```python
from build123d import *

# Parameters (mm, degrees)
CROQUIS1_W                 = 140
CROQUIS1_H                 = 140
CROQUIS1_R                 = 1.5
SALIENTE_EXTRUIR1_DEPTH    = 50
CROQUIS2_R                 = 1.75
CROQUIS2_W                 = 50
CROQUIS2_H                 = 50
CORTAR_EXTRUIR1_DEPTH      = 143
CROQUIS3_W                 = 144
CROQUIS3_H                 = 144
CROQUIS3_R                 = 1.75
CROQUIS3_W_2               = 50
CROQUIS3_H_2               = 50
SALIENTE_EXTRUIR3_DEPTH    = 50
CORTAR_EXTRUIR2_REACH      = 170.582
CORTAR_EXTRUIR3_DEPTH      = 92
CORTAR_EXTRUIR3_DEPTH_BACK = 78


with BuildPart() as part:
    # Croquis1 → Saliente-Extruir1 (new body)
    with BuildSketch(Plane(origin=(0, 0, 0), x_dir=(1, 0, 0), z_dir=(0, 1, 0))):
        Rectangle(CROQUIS1_W, CROQUIS1_H)
        with Locations(Location((-61, 61, 0), (0, 0, 270))):
            Circle(CROQUIS1_R, mode=Mode.SUBTRACT)
        with Locations(Location((66, 61, 0), (0, 0, 270))):
            Circle(CROQUIS1_R, mode=Mode.SUBTRACT)
        with Locations(Location((66, -61, 0), (0, 0, 270))):
            Circle(CROQUIS1_R, mode=Mode.SUBTRACT)
        with Locations(Location((-61, -61, 0), (0, 0, 270))):
            Circle(CROQUIS1_R, mode=Mode.SUBTRACT)
        with Locations(Location((66, 30.5, 0), (0, 0, 270))):
            Circle(CROQUIS1_R, mode=Mode.SUBTRACT)
        with Locations(Location((66, -30.5, 0), (0, 0, 270))):
            Circle(CROQUIS1_R, mode=Mode.SUBTRACT)
        with Locations(Location((-30.5, -66, 0), (0, 0, 270))):
            Circle(CROQUIS1_R, mode=Mode.SUBTRACT)
        with Locations(Location((30.5, -66, 0), (0, 0, 270))):
            Circle(CROQUIS1_R, mode=Mode.SUBTRACT)
        with Locations(Location((-30.5, 66, 0), (0, 0, 90))):
            Circle(CROQUIS1_R, mode=Mode.SUBTRACT)
        with Locations(Location((30.5, 66, 0), (0, 0, 90))):
            Circle(CROQUIS1_R, mode=Mode.SUBTRACT)
        with Locations(Location((-66, 30.5, 0), (0, 0, 90))):
            Circle(CROQUIS1_R, mode=Mode.SUBTRACT)
        with Locations(Location((-66, -30.5, 0), (0, 0, 90))):
            Circle(CROQUIS1_R, mode=Mode.SUBTRACT)
    extrude(amount=SALIENTE_EXTRUIR1_DEPTH)

    # Croquis2 → Cortar-Extruir1 (cut)
    with BuildSketch(Plane(origin=(0, 50, 0), x_dir=(1, 0, 0), z_dir=(0, 1, 0))):
        with Locations(Location((66, 61, 0), (0, 0, 270))):
            Circle(CROQUIS2_R)
        with Locations(Location((-61, 61, 0), (0, 0, 270))):
            Circle(CROQUIS2_R)
        with Locations(Location((-61, -61, 0), (0, 0, 270))):
            Circle(CROQUIS2_R)
        with Locations(Location((66, -61, 0), (0, 0, 270))):
            Circle(CROQUIS2_R)
        Polygon((-28.906513257, 63.24), (-27.313026514, 66), (-28.906513257, 68.76), (-32.093486743, 68.76), (-33.686973486, 66), (-32.093486743, 63.24), align=None)
        Polygon((32.093486743, 63.24), (33.686973486, 66), (32.093486743, 68.76), (28.906513257, 68.76), (27.313026514, 66), (28.906513257, 63.24), align=None)
        Polygon((67.593486743, 27.74), (69.186973486, 30.5), (67.593486743, 33.26), (64.406513257, 33.26), (62.813026514, 30.5), (64.406513257, 27.74), align=None)
        Polygon((67.593486743, -33.26), (69.186973486, -30.5), (67.593486743, -27.74), (64.406513257, -27.74), (62.813026514, -30.5), (64.406513257, -33.26), align=None)
        Polygon((32.093486743, -68.76), (33.686973486, -66), (32.093486743, -63.24), (28.906513257, -63.24), (27.313026514, -66), (28.906513257, -68.76), align=None)
        Polygon((-28.906513257, -68.76), (-27.313026514, -66), (-28.906513257, -63.24), (-32.093486743, -63.24), (-33.686973486, -66), (-32.093486743, -68.76), align=None)
        Polygon((-64.406513257, -33.26), (-62.813026514, -30.5), (-64.406513257, -27.74), (-67.593486743, -27.74), (-69.186973486, -30.5), (-67.593486743, -33.26), align=None)
        Polygon((-64.406513257, 27.74), (-62.813026514, 30.5), (-64.406513257, 33.26), (-67.593486743, 33.26), (-69.186973486, 30.5), (-67.593486743, 27.74), align=None)
        Rectangle(CROQUIS2_W, CROQUIS2_H)
    extrude(amount=-CORTAR_EXTRUIR1_DEPTH, mode=Mode.SUBTRACT)

    # Croquis3 → Saliente-Extruir3 (add)
    with BuildSketch(Plane(origin=(0, 50, 0), x_dir=(1, 0, 0), z_dir=(0, 1, 0))):
        Rectangle(CROQUIS3_W, CROQUIS3_H)
        with Locations(Location((-61, -61, 0), (0, 0, 270))):
            Circle(CROQUIS3_R, mode=Mode.SUBTRACT)
        with Locations(Location((-61, 61, 0), (0, 0, 270))):
            Circle(CROQUIS3_R, mode=Mode.SUBTRACT)
        with Locations(Location((66, 61, 0), (0, 0, 270))):
            Circle(CROQUIS3_R, mode=Mode.SUBTRACT)
        with Locations(Location((66, -61, 0), (0, 0, 270))):
            Circle(CROQUIS3_R, mode=Mode.SUBTRACT)
        Rectangle(CROQUIS3_W_2, CROQUIS3_H_2, mode=Mode.SUBTRACT)
        Polygon((-33.686973486, -66), (-32.093486743, -68.76), (-28.906513257, -68.76), (-27.313026514, -66), (-28.906513257, -63.24), (-32.093486743, -63.24), align=None, mode=Mode.SUBTRACT)
        Polygon((-67.593486743, -33.26), (-64.406513257, -33.26), (-62.813026514, -30.5), (-64.406513257, -27.74), (-67.593486743, -27.74), (-69.186973486, -30.5), align=None, mode=Mode.SUBTRACT)
        Polygon((28.906513257, 63.24), (32.093486743, 63.24), (33.686973486, 66), (32.093486743, 68.76), (28.906513257, 68.76), (27.313026514, 66), align=None, mode=Mode.SUBTRACT)
        Polygon((-33.686973486, 66), (-32.093486743, 63.24), (-28.906513257, 63.24), (-27.313026514, 66), (-28.906513257, 68.76), (-32.093486743, 68.76), align=None, mode=Mode.SUBTRACT)
        Polygon((62.813026514, 30.5), (64.406513257, 27.74), (67.593486743, 27.74), (69.186973486, 30.5), (67.593486743, 33.26), (64.406513257, 33.26), align=None, mode=Mode.SUBTRACT)
        Polygon((67.593486743, -33.26), (69.186973486, -30.5), (67.593486743, -27.74), (64.406513257, -27.74), (62.813026514, -30.5), (64.406513257, -33.26), align=None, mode=Mode.SUBTRACT)
        Polygon((33.686973486, -66), (32.093486743, -63.24), (28.906513257, -63.24), (27.313026514, -66), (28.906513257, -68.76), (32.093486743, -68.76), align=None, mode=Mode.SUBTRACT)
        Polygon((-64.406513257, 27.74), (-62.813026514, 30.5), (-64.406513257, 33.26), (-67.593486743, 33.26), (-69.186973486, 30.5), (-67.593486743, 27.74), align=None, mode=Mode.SUBTRACT)
    extrude(amount=-SALIENTE_EXTRUIR3_DEPTH)

    # Cortar-Extruir2: up to this face of the body (flat: up to its plane)
    cortar_extruir2_end = Plane(part.part.faces().sort_by_distance((72, 25, 0))[0])
    # Croquis4 → Cortar-Extruir2 (cut, up to the picked face)
    with BuildSketch(Plane.ZY.offset(72), mode=Mode.PRIVATE) as cortar_extruir2_sk1:
        Polygon((-25, 50), (-72, 3), (-72, 50), align=None)
    cortar_extruir2_tool1 = split(extrude(cortar_extruir2_sk1.sketch, amount=-CORTAR_EXTRUIR2_REACH, mode=Mode.PRIVATE), bisect_by=cortar_extruir2_end, keep=Keep.BOTH, mode=Mode.PRIVATE)
    # Croquis4 → Cortar-Extruir2 (cut, up to the picked face)
    with BuildSketch(Plane.ZY.offset(72), mode=Mode.PRIVATE) as cortar_extruir2_sk2:
        Polygon((72, 3), (72, 50), (25, 50), align=None)
    cortar_extruir2_tool2 = split(extrude(cortar_extruir2_sk2.sketch, amount=-CORTAR_EXTRUIR2_REACH, mode=Mode.PRIVATE), bisect_by=cortar_extruir2_end, keep=Keep.BOTH, mode=Mode.PRIVATE)
    add(cortar_extruir2_tool1.solids().sort_by(Axis((-72, 34.333333, -56.333333), (1, 0, 0)))[0], mode=Mode.SUBTRACT)
    add(cortar_extruir2_tool2.solids().sort_by(Axis((-72, 34.333333, 56.333333), (1, 0, 0)))[0], mode=Mode.SUBTRACT)

    # Croquis5 → Cortar-Extruir3 (cut, two sides: drawn at the far end of the back side and taken through both)
    with BuildSketch(Plane.XY.offset(-CORTAR_EXTRUIR3_DEPTH_BACK)):
        Polygon((-25, 50), (-72, 3), (-72, 50), align=None)
        Polygon((25, 50), (72, 3), (72, 50), align=None)
    extrude(amount=CORTAR_EXTRUIR3_DEPTH + CORTAR_EXTRUIR3_DEPTH_BACK, mode=Mode.SUBTRACT)


solid = part.part
```
Geometry: final body of the model. Coordinates: model frame, mm. A direction names the side the tool comes from. Round coordinates to 2 decimals unless told otherwise and drop trailing zeros. Loops run counter-clockwise (first coordinate to the right, second up) from the corner with the lowest first, then second, coordinate; pieces in that order, holes last. Notation, with made-up numbers: (39, -28) -> (63, -28) arc R24 ccw to (63, 2) -> close; hole circle Ø5 at (86.5, 27.25). An arc over 180 degrees is marked (long way). Write each question's results on one line, items separated by ' | '.
Item 1: Pull-direction query (Z, two-part tool) for faces 3 (the face through (64.45, 4.27, -60.19)), 4 (the face through (-1, 22, 53)), 5 (the face through (53, 22, -1)); classes: pulls with the +Z half, pulls with the -Z half, needs draft (parallel to the pull), parting line crosses it, or undercut.
Answers below:
face 3: undercut | face 4: pulls with the +Z half | face 5: needs draft
Item 2: Cut plane C-C on x = 6.5. Return the cut outline in (y, z).
Answers below:
outline: (0, -72) -> (3, -72) -> (50, -25) -> (0, -25) -> close; (0, 25) -> (50, 25) -> (3, 72) -> (0, 72) -> close
Item 3: Set-up query: faces 1 (the face through (-30, 3, -68.76)), 2 (the face through (-1, 22, -53)). Return all of +Z, -Z, +X, -X, +Y, -Y with unobstructed straight access to the full face (end or side cutting, diameter ignored); none if empty.
Answers below:
face 1: +Y, -Y | face 2: -Z, +X, -X, +Y
Item 4: Cut plane B-B on z = -6. Return the cut outline in (x, y).
Answers below:
outline: (-72, 0) -> (-25, 0) -> (-25, 50) -> (-72, 3) -> close; (25, 0) -> (72, 0) -> (72, 3) -> (25, 50) -> close
Item 5: Pin query (flat end, axial travel): pin 1 Ø10 at (x, z) = (-50.5, 45) entering from +Y; pin 2 Ø1 at (x, y) = (67, 5.5) entering from +Z; pin 3 Ø2 at (y, z) = (30.5, -39.5) entering from -X. Return the tip coordinate at first contact, or that it passes through.
Answers below:
pin 1: stops at y = 29.5 | pin 2: stops at z = 70 | pin 3: stops at x = -45.5
Item 6: Cut plane D-D on z = 56. Return the cut outline in (x, y).
Answers below:
outline: (-72, 0) -> (72, 0) -> (72, 3) -> (56, 19) -> (-56, 19) -> (-72, 3) -> close
Item 7: Cut plane A-A on y = 20. Return the cut outline in (x, z), and give its area (3 significant figures).
Answers below:
outline: (-55, -55) -> (55, -55) -> (55, 55) -> (-55, 55) -> close; hole (-25, -25) -> (25, -25) -> (25, 25) -> (-25, 25) -> close | area: 9,600 mm²
Item 8: Line query: probe 1 along Z at (x, y) = (-61, 11.75); probe 2 along Z at (x, y) = (-61, 5.5); probe 3 along Z at (x, y) = (8.5, 44.5). Output: solid intervals per line, ascending. Write a range as [from, to].
Answers below:
probe 1: z = [-63.25, -62.75], [-59.25, 59.25], [62.75, 63.25] | probe 2: z = [-69.5, -62.75], [-59.25, 59.25], [62.75, 69.5] | probe 3: z = [-30.5, -25], [25, 30.5]
